from build123d import *

# Parameters (mm, degrees)
SHAPEBINDER_W   = 20.05
SHAPEBINDER_H   = 105.775
SHAPEBINDER_R   = 6.25
PAD001_DEPTH    = 3
POCKET006_DEPTH = 3
FILLET001_R     = 0.75
SKETCH035_W     = 20
SKETCH035_H     = 1.5625
PAD015_DEPTH    = 3
POCKET025_DEPTH = 5


with BuildPart() as part:
    # ShapeBinder → Pad001 (new body)
    with BuildSketch(Plane(origin=(1.263411, 2.723963, 4.9), x_dir=(0, 1, 0), z_dir=(0, 0, 1))):
        with BuildLine():
            ThreePointArc((51.638537, 102.013411), (50.759858, 104.134731), (48.638537, 105.013411))
            Line((48.638537, 105.013411), (-54.086463, 105.013411))
            ThreePointArc((-54.086463, 105.013411), (-56.207783, 104.134731), (-57.086463, 102.013411))
            Line((-57.086463, 102.013411), (-57.086463, -99.486589))
            ThreePointArc((-57.086463, -99.486589), (-56.207783, -101.607909), (-54.086463, -102.486589))
            Line((-54.086463, -102.486589), (48.638537, -102.486589))
            ThreePointArc((48.638537, -102.486589), (50.759858, -101.607909), (51.638537, -99.486589))
            Line((51.638537, -99.486589), (51.638537, 102.013411))
        make_face()
        with Locations((-39.061463, 1.263411)):
            Rectangle(SHAPEBINDER_W, SHAPEBINDER_H, mode=Mode.SUBTRACT)
        Polygon((-44.323963, 97.013411), (32.876037, 97.013411), (32.876037, -94.486589), (-44.323963, -94.486589), (-44.323963, -55.386589), (-25.273963, -55.386589), (-25.273963, 57.913411), (-44.323963, 57.913411), align=None, mode=Mode.SUBTRACT)
        with Locations((42.257287, 89.483411)):
            Circle(SHAPEBINDER_R, mode=Mode.SUBTRACT)
        with BuildLine():
            ThreePointArc((40.257287, 73.733411), (42.257287, 75.733411), (44.257287, 73.733411))
            Line((44.257287, 73.733411), (44.257287, -62.486589))
            ThreePointArc((44.257287, -62.486589), (42.257287, -64.486589), (40.257287, -62.486589))
            Line((40.257287, -62.486589), (40.257287, 73.733411))
        make_face(mode=Mode.SUBTRACT)
        Polygon((42.257287, -72.486589), (44.757287, -74.049089), (44.757287, -75.924089), (42.257287, -77.486589), (41.319787, -77.486589), (41.319787, -76.861589), (40.538537, -77.486589), (39.757287, -76.861589), (39.757287, -75.611589), (40.538537, -76.236589), (41.319787, -75.611589), (41.319787, -74.361589), (40.538537, -73.736589), (39.757287, -74.361589), (39.757287, -73.111589), (40.538537, -72.486589), (41.319787, -73.111589), (41.319787, -72.486589), align=None, mode=Mode.SUBTRACT)
        Polygon((42.257287, -79.986589), (44.757287, -81.549089), (44.757287, -83.424089), (42.257287, -84.986589), (41.319787, -84.986589), (41.319787, -84.361589), (40.538537, -84.986589), (39.757287, -84.361589), (39.757287, -83.111589), (40.538537, -83.736589), (41.319787, -83.111589), (41.319787, -81.861589), (40.538537, -81.236589), (39.757287, -81.861589), (39.757287, -80.611589), (40.538537, -79.986589), (41.319787, -80.611589), (41.319787, -79.986589), align=None, mode=Mode.SUBTRACT)
        Polygon((42.257287, -87.486589), (44.757287, -89.049089), (44.757287, -90.924089), (42.257287, -92.486589), (41.319787, -92.486589), (41.319787, -91.861589), (40.538537, -92.486589), (39.757287, -91.861589), (39.757287, -90.611589), (40.538537, -91.236589), (41.319787, -90.611589), (41.319787, -89.361589), (40.538537, -88.736589), (39.757287, -89.361589), (39.757287, -88.111589), (40.538537, -87.486589), (41.319787, -88.111589), (41.319787, -87.486589), align=None, mode=Mode.SUBTRACT)
    extrude(amount=PAD001_DEPTH)

    # Sketch007 (on Face80 of Pad001) → Pocket006 (cut)
    with BuildSketch(Plane(origin=(0, 0, 4.9), x_dir=(1, 0, 0), z_dir=(0, 0, -1))):
        with BuildLine():
            ThreePointArc((-100.75, 56.3625), (-104.285534, 54.898034), (-105.75, 51.3625))
            Line((-105.75, -51.3625), (-105.75, 51.3625))
            ThreePointArc((-105.75, -51.3625), (-104.285534, -54.898034), (-100.75, -56.3625))
            Line((100.75, -56.3625), (-100.75, -56.3625))
            ThreePointArc((100.75, -56.3625), (104.285534, -54.898034), (105.75, -51.3625))
            Line((105.75, 51.3625), (105.75, -51.3625))
            ThreePointArc((105.75, 51.3625), (104.285534, 54.898034), (100.75, 56.3625))
            Line((-100.75, 56.3625), (100.75, 56.3625))
        make_face()
        with BuildLine():
            ThreePointArc((-100.75, 54.2125), (-102.765254, 53.377754), (-103.6, 51.3625))
            Line((-103.6, -51.3625), (-103.6, 51.3625))
            ThreePointArc((-103.6, -51.3625), (-102.765254, -53.377754), (-100.75, -54.2125))
            Line((100.75, -54.2125), (-100.75, -54.2125))
            ThreePointArc((100.75, -54.2125), (102.765254, -53.377754), (103.6, -51.3625))
            Line((103.6, 51.3625), (103.6, -51.3625))
            ThreePointArc((103.6, 51.3625), (102.765254, 53.377754), (100.75, 54.2125))
            Line((-100.75, 54.2125), (100.75, 54.2125))
        make_face(mode=Mode.SUBTRACT)
    extrude(amount=-POCKET006_DEPTH, mode=Mode.SUBTRACT)

    # Fillet001
    fillet001_edges = [part.edges().sort_by_distance(p)[0] for p in [
        (-95.75, 35.6, 6.4),
        (-95.75, -41.6, 6.4),
        (-56.65, -22.55, 6.4),
        (-56.65, -41.6, 6.4),
        (-52.8875, -46.3625, 6.4),
        (52.8875, -46.3625, 6.4),
        (52.8875, -26.3125, 6.4),
        (95.75, 35.6, 6.4),
        (-52.8875, -26.3125, 6.4),
        (95.75, -41.6, 6.4),
        (56.65, -22.55, 6.4),
        (56.65, -41.6, 6.4),
    ]]
    fillet(fillet001_edges, radius=FILLET001_R)

    # Sketch035 (on Face93 of Fillet001) → Pad015 (join)
    with BuildSketch(Plane.XY.offset(7.9)):
        with Locations((83.75, 43.2625)):
            Rectangle(SKETCH035_W, SKETCH035_H)
    extrude(amount=-PAD015_DEPTH)

    # Sketch036 (on Face69 of Pad015) → Pocket025 (cut)
    with BuildSketch(Plane.XY.offset(7.9)):
        Polygon((73.75, 44.04375), (73.35, 43.2625), (73.75, 42.48125), (75.25, 42.48125), (74.85, 43.2625), (75.25, 44.04375), align=None)
        Polygon((78.75, 44.04375), (79.15, 43.2625), (78.75, 42.48125), (77.25, 42.48125), (77.65, 43.2625), (77.25, 44.04375), align=None)
        Polygon((81.25, 44.04375), (80.85, 43.2625), (81.25, 42.48125), (82.75, 42.48125), (82.35, 43.2625), (82.75, 44.04375), align=None)
        Polygon((86.25, 44.04375), (86.65, 43.2625), (86.25, 42.48125), (84.75, 42.48125), (85.15, 43.2625), (84.75, 44.04375), align=None)
        Polygon((88.75, 44.04375), (88.35, 43.2625), (88.75, 42.48125), (90.25, 42.48125), (89.85, 43.2625), (90.25, 44.04375), align=None)
        Polygon((93.75, 44.04375), (92.25, 44.04375), (92.65, 43.2625), (92.25, 42.48125), (93.75, 42.48125), (94.15, 43.2625), align=None)
    extrude(amount=-POCKET025_DEPTH, mode=Mode.SUBTRACT)


solid = part.part
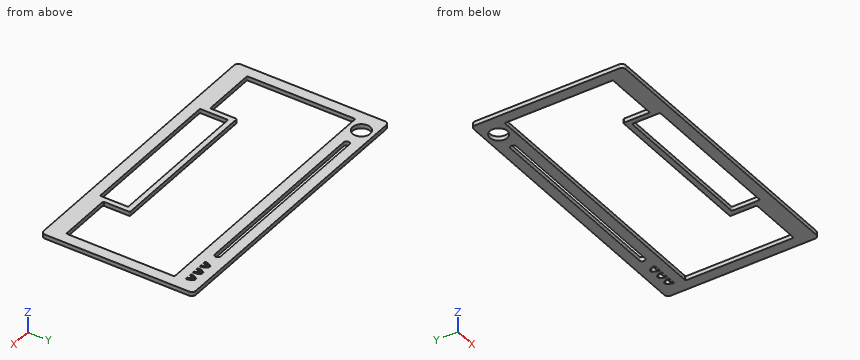
For this review, take the finished solid that the model builds, in its own axes (mm). Coordinates: 2 decimals unless noted, no trailing zeros. Order: outer loops, then holes, each group sorted by start corner. A loop starts at its lowest first (then second) coordinate and runs counter-clockwise, first axis right, second up. Notation, with made-up numbers: (7, 8.25) - (38, 8.25) arc R25 ccw to (38, 36.25) - close; hole circle Ø8 at (-36, 71.25). An arc over 180 degrees is marked (long way). Use one line per item in the form item = value.
Q1. For probe 1 along Y at (x, z) = (84.5, 5); probe 2 along Y at (x, z) = (-88.22, 5.8); probe 3 along X at (y, z) = (-31, 5.95), list the stretches that pass through material, from the lowest coordinate up. Write a range as from..to.
Checked values:
probe_1 = -54.21..-41.6, 35.6..44.04, 47.48..54.21
probe_2 = -54.21..-41.6, 35.6..38.73, 51.23..54.21
probe_3 = -103.6..-95.75, -56.65..-52.89, 52.89..56.65, 95.75..103.6
Q2. Consider section B-B (x = -88.22). Give the boundary of the cut face in (y, z).
Checked values:
outline = (-54.21, 4.9) - (-41.6, 4.9) - (-41.6, 7.9) - (-54.21, 7.9) - close; (35.6, 4.9) - (38.73, 4.9) - (38.73, 7.9) - (35.6, 7.9) - close; (51.23, 4.9) - (54.21, 4.9) - (54.21, 7.9) - (51.23, 7.9) - close
Q3. Consider section D-D (z = 6.3). Give the number of separate pieces and of enclosed holes in the cut face, then the cut area to 3 significant figures.
Checked values:
separate_pieces = 1
enclosed_holes = 7
area = 6,980 mm2
Q4. Consider section C-C (y = 1.5). Give the boundary of the cut face in (x, z), then the cut area to 3 significant figures.
Checked values:
outline = (-103.6, 4.9) - (-95.75, 4.9) - (-95.75, 7.9) - (-103.6, 7.9) - close; (95.75, 4.9) - (103.6, 4.9) - (103.6, 7.9) - (95.75, 7.9) - close
area = 47.1 mm2
Q5. Consider section A-A (x = -32). Give the boundary of the cut face in (y, z), then the cut area to 3 significant figures.
Checked values:
outline = (-54.21, 4.9) - (-46.36, 4.9) - (-46.36, 7.9) - (-54.21, 7.9) - close; (-26.31, 4.9) - (-22.55, 4.9) - (-22.55, 7.9) - (-26.31, 7.9) - close; (35.6, 4.9) - (42.98, 4.9) - (42.98, 7.9) - (35.6, 7.9) - close; (46.98, 4.9) - (54.21, 4.9) - (54.21, 7.9) - (46.98, 7.9) - close
area = 78.7 mm2
